Input: part model. Units: mm. Frame: model coordinates. A direction names the side the tool comes from. Round coordinates to 2 decimals unless told otherwise and drop trailing zeros. Order: outer loops, then holes, each group sorted by start corner. A loop starts at its lowest first (then second) coordinate and runs counter-clockwise, first axis right, second up. Notation, with made-up numbers: (-12.5, -19.75) -> (46.5, -19.75) arc R24 cw to (46.5, -5.75) -> close; hole circle Ø7 at (17.5, 20.5). An arc over 180 degrees is marked (long way). Use a Markdown table: item, result.
Autodesk Inventor part; units mm, degrees
ref_plane "YZ Plane" through (0, 0, 0) normal (1, 0, 0) x (0, 1, 0)
ref_plane "XZ Plane" through (0, 0, 0) normal (0, 1, 0) x (-1, 0, 0)
ref_plane "XY Plane" through (0, 0, 0) normal (0, 0, 1) x (1, 0, 0)
sketch "Sketch1" plane through (0, 0, 0) normal (0, 0, 1) x (1, 0, 0)
  circle A0 centre (0, 0) radius 6.5
  circle A1 centre (0, 0) radius 5
  circle A2 centre (0, 0) radius 1.5
  dimension "d11" = 13
  dimension "d12" = 10
  dimension "d13" = 3
extrude "Extrusion1" add sketch "Sketch1" along normal blind 27 contours A0 | A1
extrude "Extrusion3" add sketch "Sketch1" against normal blind 6 contours A1
extrude "Extrusion4" add sketch "Sketch1" against normal blind 13 contours A2
sketch "Sketch3" plane through (0, 0, -13) normal (0, 0, -1) x (-1, 0, 0)
  circle A0 centre (0, 0) radius 1
  dimension "d18" = 2
extrude "Extrusion5" add sketch "Sketch3" along normal blind 6
properties part number "Solinoid"
1) Set-up query: faces 1 (the face through (0, 2, 27)), 2 (the face through (2, -5, 0)), 3 (the face through (0, 0, 0)). Return all of +Z, -Z, +X, -X, +Y, -Y with unobstructed straight access to the full face (end or side cutting, diameter ignored); none if empty.
Answer key:
| item | result |
|---|---|
| face 1 | +Z, +X, -X, +Y, -Y |
| face 2 | -Z |
| face 3 | +Z |
2) Draft query along X for faces 4 (the face through (-1.5, -0.07, 13.31)), 5 (the face through (-1.2, 1.2, -6)), 6 (the face through (-5.158, 3.955, 13.311)). Return one class per face: released by +X, released by -X, zero draft, split by the parting line, or undercut.
Answer key:
| item | result |
|---|---|
| face 4 | undercut |
| face 5 | zero draft |
| face 6 | split by the parting line |
3) Cut plane A-A on x = 0. Return loops of the section in (y, z), and give its area (3 significant figures).
Answer key:
| item | result |
|---|---|
| outline | (-6.5, 0) -> (-5, 0) -> (-5, -6) -> (-1.5, -6) -> (-1.5, -13) -> (-1, -13) -> (-1, -19) -> (1, -19) -> (1, -13) -> (1.5, -13) -> (1.5, -6) -> (5, -6) -> (5, 0) -> (6.5, 0) -> (6.5, 27) -> (1.5, 27) -> (1.5, 0) -> (-1.5, 0) -> (-1.5, 27) -> (-6.5, 27) -> close |
| area | 363 mm^2 |
4) Cut plane D-D on z = -7. Return loops of the section in (x, y), and give its area (3 significant figures).
Answer key:
| item | result |
|---|---|
| outline | circle Ø3 at (0, 0) |
| area | 7.07 mm^2 |
5) Ray query, probe 1 along Y at (x, z) = (0, 14); probe 2 along Z at (x, y) = (0.25, 2.5); probe 3 along X at (y, z) = (0.25, 17.5). Return the intervals inside material, ascending.
Answer key:
| item | result |
|---|---|
| probe 1 | y = -6.5 to -1.5, 1.5 to 6.5 |
| probe 2 | z = -6 to 27 |
| probe 3 | x = -6.5 to -1.48, 1.48 to 6.5 |
6) Contact query for flat-ended pins moving along their axis: P1, Ø3, axis at y = -2.5, z = 5, coming from the -X side; P2, Ø0.9, axis at x = 0, y = 0.5, coming from the +Z side; P3, Ø5, axis at x = -1.5, z = -13, coming from the -Y side. Output: stop coordinate, or through.
Answer key:
| item | result |
|---|---|
| P1 | stops at x = -6.42 |
| P2 | stops at z = 0 |
| P3 | stops at y = -1.5 |
7) Cut plane C-C on z = 23.5. Return loops of the section in (x, y).
Answer key:
| item | result |
|---|---|
| outline | circle Ø13 at (0, 0); hole circle Ø3 at (0, 0) |
